Source: CAD feature listing. Evaluate the final solid. Frame: model axes, mm. A direction names the side the tool comes from. Give positions to 0.01 mm unless a question says otherwise; leave off trailing zeros. Order: outer loops, then holes, each group sorted by start corner. A loop starts at its lowest first (then second) coordinate and runs counter-clockwise, first axis right, second up.
from build123d import *

# Parameters (mm, degrees)
F0_W      = 618.75
F0_H      = 833.4375
F1_DEPTH  = 190.5
F2_W      = 567.95
F2_H      = 139.7
F3_DEPTH  = 833.4385
F4_W      = 567.95
F4_H      = 782.6375
F5_DEPTH  = 190.501
F6_W      = 139.7
F6_H      = 782.6375
F7_DEPTH  = 618.751
F8_W      = 25.4
F8_H      = 25.4
F9_DEPTH  = 787.4
F10_W     = 25.4
F10_H     = 25.4
F11_DEPTH = 787.4
F12_W     = 25.4
F12_H     = 25.4
F13_DEPTH = 787.4
F14_W     = 25.4
F14_H     = 25.4
F15_DEPTH = 787.4
F16_W     = 25.4
F16_H     = 25.4
F17_DEPTH = 313.95
F18_W     = 313.95
F18_H     = 25.4
F19_DEPTH = 25.4


with BuildPart() as f1:
    # F0 (on Front) → F1 (new body)
    with BuildSketch(Plane.XZ):
        with Locations((-19.982701, 279.260447)):
            Rectangle(F0_W, F0_H)
    extrude(amount=F1_DEPTH)

    # F2 (on face) → F3 (cut, through all)
    with BuildSketch(Plane.XY.offset(695.979197)):
        with Locations((-19.982701, -95.25)):
            Rectangle(F2_W, F2_H)
    extrude(amount=-F3_DEPTH, mode=Mode.SUBTRACT)

    # F4 (on face) → F5 (cut, through all)
    with BuildSketch(Plane(origin=(0, 0, 0), x_dir=(-1, 0, 0), z_dir=(0, 1, 0))):
        with Locations((19.982701, 279.260447)):
            Rectangle(F4_W, F4_H)
    extrude(amount=-F5_DEPTH, mode=Mode.SUBTRACT)

    # F6 (on face) → F7 (cut, through all)
    with BuildSketch(Plane.YZ.offset(289.392299)):
        with Locations((-95.25, 279.260447)):
            Rectangle(F6_W, F6_H)
    extrude(amount=-F7_DEPTH, mode=Mode.SUBTRACT)

    # F8 (on face) → F9 (join)
    with BuildSketch(Plane(origin=(0, 0, 670.579197), x_dir=(1, 0, 0), z_dir=(0, 0, -1))):
        with Locations((149.692299, 177.8)):
            Rectangle(F8_W, F8_H)
    extrude(amount=F9_DEPTH)

    # F10 (on face) → F11 (join)
    with BuildSketch(Plane(origin=(0, 0, 670.579197), x_dir=(1, 0, 0), z_dir=(0, 0, -1))):
        with Locations((-189.657701, 177.8)):
            Rectangle(F10_W, F10_H)
    extrude(amount=F11_DEPTH)

    # F12 (on face) → F13 (join)
    with BuildSketch(Plane(origin=(0, 0, 670.579197), x_dir=(1, 0, 0), z_dir=(0, 0, -1))):
        with Locations((-189.657701, 12.7)):
            Rectangle(F12_W, F12_H)
    extrude(amount=F13_DEPTH)

    # F14 (on face) → F15 (join)
    with BuildSketch(Plane(origin=(0, 0, 670.579197), x_dir=(1, 0, 0), z_dir=(0, 0, -1))):
        with Locations((149.692299, 12.7)):
            Rectangle(F14_W, F14_H)
    extrude(amount=F15_DEPTH)

    # F16 (on face) → F17 (join, through all)
    with BuildSketch(Plane.YZ.offset(-176.957701)):
        with Locations((-177.8, 607.079197)):
            Rectangle(F16_W, F16_H)
    extrude(amount=F17_DEPTH)

    # F18 (on face) → F19 (cut, through all)
    with BuildSketch(Plane.XZ.offset(190.5)):
        with Locations((-19.982701, 683.279197)):
            Rectangle(F18_W, F18_H)
    extrude(amount=-F19_DEPTH, mode=Mode.SUBTRACT)


solid = f1.part
1) First-contact query: pin 1 Ø7.5 at (x, z) = (-322, 98) entering from +Y; pin 2 Ø4 at (y, z) = (-29, 308.5) entering from -X. Flat tips, straight axial feed; report the tip coordinate or a pass-through.
Checks:
pin 1: stops at y = 0
pin 2: passes through
2) Section query A-A on y = -93. Output: boundary loops of the cut face in (x, z).
Checks:
outline: (-329.36, -137.46) - (-303.96, -137.46) - (-303.96, -112.06) - (-329.36, -112.06) - close; (-329.36, 670.58) - (-303.96, 670.58) - (-303.96, 695.98) - (-329.36, 695.98) - close; (263.99, -137.46) - (289.39, -137.46) - (289.39, -112.06) - (263.99, -112.06) - close; (263.99, 670.58) - (289.39, 670.58) - (289.39, 695.98) - (263.99, 695.98) - close
3) Pull-direction query (X, two-part tool) for faces 5 (the face through (162.392, -13, 285)), 6 (the face through (-22, -178, 594.379)), 7 (the face through (139, -190.5, 219)); classes: +X half, -X half, draft (parallel to the pull), parting line (faces both ways), or undercut.
Checks:
face 5: undercut
face 6: undercut
face 7: draft
4) Section query B-B on z = 465. State how many separate pieces and enclosed holes the cut face has, and give its area (3 significant figures).
Checks:
separate pieces: 8
enclosed holes: 0
area: 5,160 mm2
5) Section query D-D on y = -12. Output: boundary loops of the cut face in (x, z), and give its area (3 significant figures).
Checks:
outline: (-329.36, -137.46) - (289.39, -137.46) - (289.39, 695.98) - (-329.36, 695.98) - close; hole (-303.96, -112.06) - (-202.36, -112.06) - (-202.36, 670.58) - (-303.96, 670.58) - close; hole (-176.96, -112.06) - (136.99, -112.06) - (136.99, 670.58) - (-176.96, 670.58) - close; hole (162.39, -112.06) - (263.99, -112.06) - (263.99, 670.58) - (162.39, 670.58) - close
area: 111,000 mm2
6) Reachability of faces 1 (the face through (277, -165.1, 274)), 2 (the face through (-21, -24, -137.458)), 3 (the face through (-190, -25.4, 281)), 4 (the face through (214, -13, 670.579)) from +Z, -Z, +X, -X, +Y, -Y: full face, straight path, thin tool, end or side. Return the list, or none.
Checks:
face 1: +X, -X
face 2: -Z, +X, -X, +Y, -Y
face 3: +Z, -Z
face 4: +Y, -Y
7) Ray query, L1, parallel to X at y = -24, z = 312; L2, parallel to Z at x = 178.5, y = -175.5. Return the intervals inside material, ascending.
Checks:
L1: x = -329.36 to -303.96, -202.36 to -176.96, 136.99 to 162.39, 263.99 to 289.39
L2: z = -137.46 to -112.06, 670.58 to 695.98
8) Section query C-C on x = -163. Output: boundary loops of the cut face in (y, z), and give its area (3 significant figures).
Checks:
outline: (-190.5, -137.46) - (-165.1, -137.46) - (-165.1, -112.06) - (-190.5, -112.06) - close; (-190.5, 594.38) - (-165.1, 594.38) - (-165.1, 619.78) - (-190.5, 619.78) - close; (-25.4, -137.46) - (0, -137.46) - (0, -112.06) - (-25.4, -112.06) - close; (-25.4, 670.58) - (0, 670.58) - (0, 695.98) - (-25.4, 695.98) - close
area: 2,580 mm2
